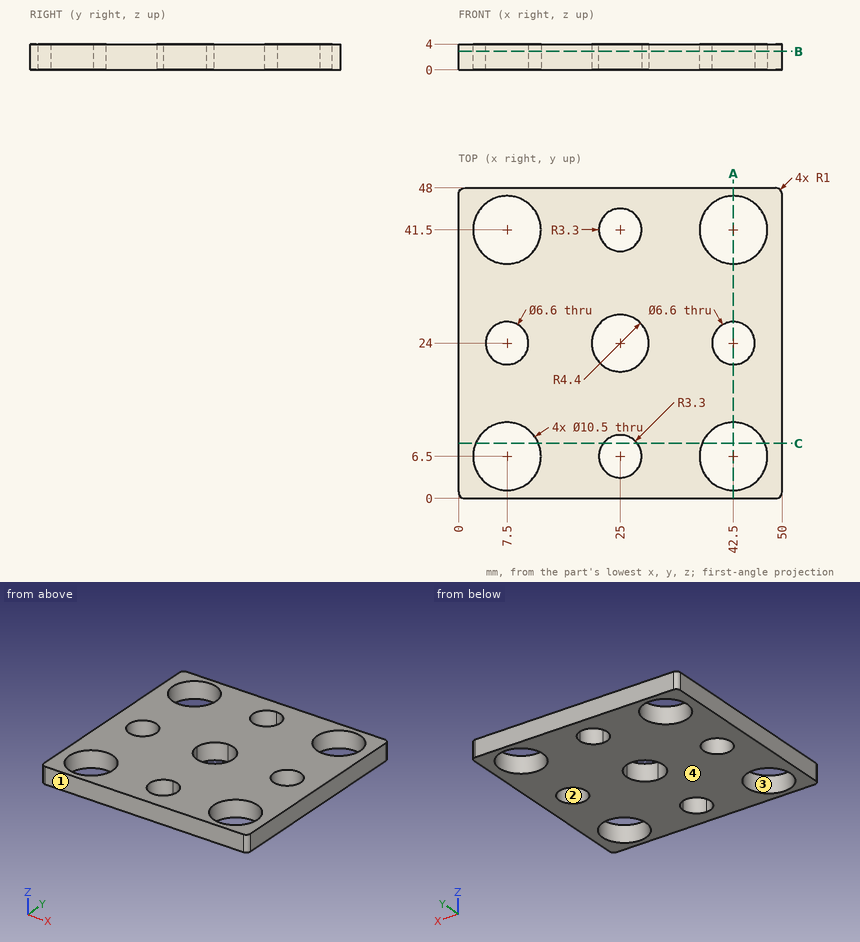
Geometry check sheet. Reference: drawing and pictorial views, mm from the part's lowest x, y, z. Round coordinates to 2 decimals unless told otherwise and drop trailing zeros. Order: outer loops, then holes, each group sorted by start corner. A loop starts at its lowest first (then second) coordinate and runs counter-clockwise, first axis right, second up. Notation, with made-up numbers: M 33.25,50 L 71.25,50 A12 ccw 71.25,64 Z; hole C -7.75,24.5 d4. An arc over 180 degrees is marked long. Write item = value, one per line.
Q1. Section check B-B (z = 2.85). Give the number of separate pieces and of enclosed holes in the cut face, plus the area to 3 significant figures.
Answer block:
separate_pieces = 1
enclosed_holes = 9
area = 1,860 mm^2
Q2. Scan lines: line 1 (Y direction, x = 42.5, z = 1.85); line 2 (Y direction, x = 12, z = 3); line 3 (X direction, y = 42.5, z = 2.6). Record each from-to range of solid material in increasing order.
Answer block:
line_1 = 0 to 1.25, 11.75 to 20.7, 27.3 to 36.25, 46.75 to 48
line_2 = 0 to 3.8, 9.2 to 38.8, 44.2 to 48
line_3 = 0 to 2.35, 12.65 to 21.86, 28.14 to 37.35, 47.65 to 50
Q3. Release check for a two-part mould opening along Y. For the marked faces 1, 2, 3 and 4 record: released by +Y, released by -Y, zero draft, split by the parting line, or undercut.
Answer block:
face_1 = released by -Y
face_2 = undercut
face_3 = undercut
face_4 = zero draft
Q4. Section check A-A (x = 42.5). Enter the section's corners in (y, z), plus the area to 3 significant figures.
Answer block:
outline = M 0,0 L 1.25,0 L 1.25,4 L 0,4 Z; M 11.75,0 L 20.7,0 L 20.7,4 L 11.75,4 Z; M 27.3,0 L 36.25,0 L 36.25,4 L 27.3,4 Z; M 46.75,0 L 48,0 L 48,4 L 46.75,4 Z
area = 81.6 mm^2
Q5. Section check C-C (y = 8.5). Enter the section's corners in (x, z).
Answer block:
outline = M 0,0 L 2.65,0 L 2.65,4 L 0,4 Z; M 12.35,0 L 22.38,0 L 22.38,4 L 12.35,4 Z; M 27.62,0 L 37.65,0 L 37.65,4 L 27.62,4 Z; M 47.35,0 L 50,0 L 50,4 L 47.35,4 Z
